from build123d import *

# Parameters (mm, degrees)
F2_W     = 0.591972
F2_H     = 6.072902
F3_DEPTH = 1


with BuildPart() as f1:
    # F0 (on Front) → F1 (revolve)
    with BuildSketch(Plane.XZ):
        Polygon((0, 2.6), (0, 0), (10, 0), (10, 1.5), (1.1, 1.5), align=None)
    revolve(axis=Axis((5, 0, 0), (-1, 0, 0)))

    # F2 (on face) → F3 (cut)
    with BuildSketch(Plane(origin=(0, 0, 0), x_dir=(0, -1, 0), z_dir=(-1, 0, 0))):
        Rectangle(F2_W, F2_H)
    extrude(amount=-F3_DEPTH, mode=Mode.SUBTRACT)


solid = f1.part
Geometry: final body of the model. Coordinates: model frame, mm. A direction names the side the tool comes from. Give positions to 0.01 mm unless a question says otherwise; leave off trailing zeros. Write each loop counter-clockwise with the first axis right and the second up, starting at its lowest first coordinate (ties: lowest second). Pieces come first, ordered by that corner, then holes.
(1) Cut plane A-A, the plane z = 0. Return loops of the section in (x, y).
(2) Cut plane B-B, the plane y = 0. Return loops of the section in (x, z).
(3) Ray query, line 1 (X direction, y = 0.2, z = -1.45); line 2 (Y direction, x = 3.75, z = 0). Return the intervals inside material, ascending.
(4) Mould query, pull axis Y, two halves, no side actions, for faces 1 (the flat face through (0, 1, 0)), 2 (the flat face through (0.5, 0.296, 0)), 3 (the conical face through (0.91, -0.65, 1.56)). Classes: released by +Y, released by -Y, zero draft, split by the parting line, or undercut.
(5) Access query for faces 4 (the flat face through (10, 0, 0)), 5 (the flat face through (0.5, -0.296, 0)), 6 (the cylindrical face through (5.49, 0.07, -1.5)). Directions: +Z, -Z, +X, -X, +Y, -Y. A direction counts if a zero-diameter tool reaches every point of the face in a straight line with its end or side. Return the directions, or none.
(6) Cut plane C-C, the plane x = 1.75. Return loops of the section in (y, z), then the cut area to 3 significant figures.
(7) First-contact query: P1, Ø0.8, axis at x = 0.5, z = -0.5, coming from the +Y side; P2, Ø3, axis at y = 0.5, z = -0.5, coming from the -X side; P3, Ø0.5, axis at x = 0.5, z = -0.5, coming from the -Y side; P4, Ø2, axis at x = 5, z = 0, coming from the +Y side. Flat tips, straight axial feed; report the tip coordinate or a pass-through.
Values follow:
1. outline: (0, -2.6) - (1.1, -1.5) - (10, -1.5) - (10, 1.5) - (1.1, 1.5) - (0, 2.6) - (0, 0.3) - (1, 0.3) - (1, -0.3) - (0, -0.3) - close
2. outline: (1, -1.6) - (1.1, -1.5) - (10, -1.5) - (10, 1.5) - (1.1, 1.5) - (1, 1.6) - close
3. line 1: x = 1 to 10
3. line 2: y = -1.5 to 1.5
4. face 1: zero draft
4. face 2: undercut
4. face 3: split by the parting line
5. face 4: +Z, -Z, +X, +Y, -Y
5. face 5: +Z, -Z, -X
5. face 6: +X
6. outline: circle Ø3 at (0, 0)
6. area: 7.07 mm2
7. P1: stops at y = 2.46
7. P2: stops at x = 0
7. P3: stops at y = -2.3
7. P4: stops at y = 1.5
